Build history of the part. All positions in model axes, mm. A direction names the side the tool comes from. Give positions to 0.01 mm unless a question says otherwise; leave off trailing zeros. Write each loop counter-clockwise with the first axis right and the second up, starting at its lowest first coordinate (ties: lowest second). Pieces come first, ordered by that corner, then holes. Notation, with made-up numbers: M -34,-16 L 19,-16 A16 cw 19,0 Z; hole C -37.5,0 d10. An arc over 180 degrees is marked long. One line per item, written item: value. Start each with the question number.
from build123d import *

# Parameters (mm, degrees)
CYLINDER_R     = 1.9
CYLINDER_DEPTH = 10
BOX_W          = 10
BOX_H          = 10
BOX_DEPTH      = 3
FILLET_R       = 4
BOX001_W       = 2
BOX001_H       = 30
BOX001_DEPTH   = 10
FILLET001_R    = 2


with BuildPart() as hole:
    # Cylinder → Cylinder (new body)
    with BuildSketch(Plane.XY):
        Circle(CYLINDER_R)
    extrude(amount=CYLINDER_DEPTH)


with BuildPart() as bottom_fillet:
    # Box → Box (new body)
    with BuildSketch(Plane(origin=(-5, -5, 0), x_dir=(1, 0, 0), z_dir=(0, 0, 1))):
        with Locations((5, 5)):
            Rectangle(BOX_W, BOX_H)
    extrude(amount=BOX_DEPTH)

    # Fillet
    fillet_edges = [bottom_fillet.edges().sort_by_distance(p)[0] for p in [
        (5, -5, 1.5),
        (5, 5, 1.5),
    ]]
    fillet(fillet_edges, radius=FILLET_R)


with BuildPart() as lock_cut:
    # Box001 → Box001 (new body)
    with BuildSketch(Plane(origin=(-7, -8, -5), x_dir=(1, 0, 0), z_dir=(0, 0, 1))):
        with Locations((1, 15)):
            Rectangle(BOX001_W, BOX001_H)
    extrude(amount=BOX001_DEPTH)

    # Fillet001
    fillet001_edges = [lock_cut.edges().sort_by_distance(p)[0] for p in [
        (-6, -8, -5),
        (-6, -8, 5),
        (-6, 22, -5),
        (-6, 22, 5),
    ]]
    fillet(fillet001_edges, radius=FILLET001_R)

    # Fusion: union bottom fillet
    add(bottom_fillet.part)

    # Cut: cut hole
    add(hole.part, mode=Mode.SUBTRACT)


solid = lock_cut.part
1) Band-saw the part on A-A (x = 0). List the corners of the cut face in (y, z).
2) Mould opens along X. For faces 5 (the face through (3.797, -3.859, 1.521)), 6 (the face through (-2.3, 0.1, 0)), 7 (the face through (-1.9, 0.08, 1.48)) say: released by +X, released by -X, zero draft, split by the parting line, or undercut.
3) Probe line 1 along Y through (x, z) = (0, 1.55); line 2 along X through (y, z) = (0, 0.8); line 3 along Y through (x, z) = (-3.5, 2.5). List the from-to ranges inside material, lowest first. Write a range as from..to.
4) Band-saw the part on C-C (z = 1). List the corners of the cut face in (x, y).
5) Band-saw the part on B-B (y = 0). List the corners of the cut face in (x, z).
6) Drop flat-ended pins along their axis: P1, Ø5, axis at x = -2, z = 3.5, coming from the +Y side; P2, Ø6, axis at x = 2.5, z = 2.5, coming from the -Y side; P3, Ø2, axis at x = 3, z = 0, coming from the -Y side; P4, Ø1.5, axis at x = 0.5, y = 7, coming from the -Z side. Give the stop position or say it passes through.
7) Band-saw the part on D-D (x = -2.5). List the corners of the cut face in (y, z), then the cut area to 3 significant figures.
8) Tool access for faces 1 (the face through (5, 0, 1)), 2 (the face through (-2, -5, 1)), 3 (the face through (-2, 5, 1)), 4 (the face through (-2.3, 0.1, 3)): list every direction of +Z, -Z, +X, -X, +Y, -Y with a clear straight run to the whole face (end or side of a thin tool).
Model answer:
1. outline: M -5,0 L -1.9,0 L -1.9,3 L -5,3 Z; M 1.9,0 L 5,0 L 5,3 L 1.9,3 Z
2. face 5: released by +X
2. face 6: zero draft
2. face 7: undercut
3. line 1: y = -5..-1.9, 1.9..5
3. line 2: x = -7..-1.9, 1.9..5
3. line 3: y = -5..5
4. outline: M -7,-8 L -5,-8 L -5,-5 L 1,-5 A4 ccw 5,-1 L 5,1 A4 ccw 1,5 L -5,5 L -5,22 L -7,22 Z; hole C 0,0 d3.8
5. outline: M -7,-5 L -5,-5 L -5,0 L -1.9,0 L -1.9,3 L -5,3 L -5,5 L -7,5 Z; M 1.9,0 L 5,0 L 5,3 L 1.9,3 Z
6. P1: stops at y = 5
6. P2: stops at y = -5
6. P3: stops at y = -4.87
6. P4: passes through
7. outline: M -5,0 L 5,0 L 5,3 L -5,3 Z
7. area: 30.0 mm²
8. face 1: +Z, -Z, +X, +Y, -Y
8. face 2: +Z, -Z, +X, -Y
8. face 3: +Z, -Z, +X, +Y
8. face 4: +Z, +X, +Y, -Y
